from build123d import *

# Parameters (mm, degrees)
BOSS_EXTRUDE1_DEPTH = 10
SKETCH2_R           = 2
CUT_EXTRUDE1_DEPTH  = 22.973952412


with BuildPart() as part:
    # Sketch1 → Boss-Extrude1 (new body)
    with BuildSketch(Plane(origin=(0, 0, 0), x_dir=(1, 0, 0), z_dir=(0, 1, 0))):
        with BuildLine():
            Line((-5.941155294, 12.923797457), (-5.941155294, 6.423797457))
            ThreePointArc((-5.941155294, 6.423797457), (0, -8.75), (5.941155294, 6.423797457))
            Line((5.941155294, 6.423797457), (5.941155294, 12.923797457))
            Line((5.941155294, 12.923797457), (3.441155294, 12.923797457))
            Line((3.441155294, 12.923797457), (3.441155294, 8.044933203))
            Line((3.441155294, 8.044933203), (3.441155294, 6.381296909))
            ThreePointArc((3.441155294, 6.381296909), (6.22538657, 3.715785524), (7.25, 0))
            ThreePointArc((7.25, 0), (-3.715785524, -6.22538657), (-3.441155294, 6.381296909))
            Line((-3.441155294, 6.381296909), (-3.441155294, 8.044933203))
            Line((-3.441155294, 8.044933203), (-3.441155294, 12.923797457))
            Line((-3.441155294, 12.923797457), (-5.941155294, 12.923797457))
        make_face()
    extrude(amount=BOSS_EXTRUDE1_DEPTH)

    # Sketch2 → Cut-Extrude1 (cut, through all)
    with BuildSketch(Plane(origin=(5.941155294, 0, 0), x_dir=(0, 0, -1), z_dir=(1, 0, 0))):
        with Locations((9.673797457, 5)):
            Circle(SKETCH2_R)
    extrude(amount=-CUT_EXTRUDE1_DEPTH, mode=Mode.SUBTRACT)


solid = part.part
Part model, mm, in its own coordinate system. A direction names the side the tool comes from. Give positions to 0.01 mm unless a question says otherwise; leave off trailing zeros. Order: outer loops, then holes, each group sorted by start corner. A loop starts at its lowest first (then second) coordinate and runs counter-clockwise, first axis right, second up. Notation, with made-up numbers: (59.25, 17.5) - (102.25, 17.5) arc R21 cw to (102.25, 38.5) - close; hole circle Ø9 at (15, -25.75). An arc over 180 degrees is marked (long way). One line per question, with ' | ' between items.
1. Band-saw the part on A-A on x = -5.25. List the corners of the cut face in (y, z), then the cut area to 3 significant figures.
Filled in:
outline: (0, -12.92) - (10, -12.92) - (10, -5) - (0, -5) - close; (0, 5) - (10, 5) - (10, 7) - (0, 7) - close; hole circle Ø4 at (5, -9.67) | area: 86.7 mm²
2. Band-saw the part on B-B on y = 5. List the corners of the cut face in (x, z).
Filled in:
outline: (-5.94, -12.92) - (-3.44, -12.92) - (-3.44, -11.67) - (-5.94, -11.67) - close; (-5.94, -7.67) - (-3.44, -7.67) - (-3.44, -6.38) arc R7.25 cw (long way) to (3.44, -6.38) - (3.44, -7.67) - (5.94, -7.67) - (5.94, -6.42) arc R8.75 ccw (long way) to (-5.94, -6.42) - close; (3.44, -12.92) - (5.94, -12.92) - (5.94, -11.67) - (3.44, -11.67) - close
3. Drop flat-ended pins along their axis: P1, Ø5, axis at y = 5, z = -9.67, coming from the +X side; P2, Ø2, axis at y = 1, z = -6, coming from the +X side; P3, Ø2, axis at y = 4, z = -10, coming from the -X side. Give the stop position or say it passes through.
Filled in:
P1: x = 5.94 | P2: x = 7.18 | P3: x = -5.94
4. Band-saw the part on C-C on z = -10.5. List the corners of the cut face in (x, y), then the cut area to 3 significant figures.
Filled in:
outline: (-5.94, 0) - (-3.44, 0) - (-3.44, 3.18) - (-5.94, 3.18) - close; (-5.94, 6.82) - (-3.44, 6.82) - (-3.44, 10) - (-5.94, 10) - close; (3.44, 0) - (5.94, 0) - (5.94, 3.18) - (3.44, 3.18) - close; (3.44, 6.82) - (5.94, 6.82) - (5.94, 10) - (3.44, 10) - close | area: 31.8 mm²
5. Pull direction Y, two halves, no side cores. Call faces 1 (the face through (-4.674, 6.983, -9.413)), 2 (the face through (-5, 0, -6)), 3 (the face through (-5, 10, -6)): +Y half, -Y half, draft (parallel to the pull), parting line (faces both ways), or undercut.
Filled in:
face 1: undercut | face 2: -Y half | face 3: +Y half
6. Band-saw the part on D-D on x = -7. List the corners of the cut face in (y, z).
Filled in:
outline: (0, -5.25) - (10, -5.25) - (10, -1.89) - (0, -1.89) - close; (0, 1.89) - (10, 1.89) - (10, 5.25) - (0, 5.25) - close
7. Which spindle directions (+Z, -Z, +X, -X, +Y, -Y) get a long thin tool onto all of the face, cutting with end or side? Do faces 4 (the face through (5.941, 5, -7)), 5 (the face through (-5.941, 5, -12)), 6 (the face through (-3.441, 5, -12)), 7 (the face through (-5, 5, -12.924)). Say none if no direction does.
Filled in:
face 4: -Z, +X, +Y, -Y | face 5: -Z, -X, +Y, -Y | face 6: -Z, +Y, -Y | face 7: -Z, +X, -X, +Y, -Y
8. Drill centre lines: probe 1 along X at (y, z) = (3.5, 0); probe 2 along X at (y, z) = (2, -8.25); probe 3 along Z at (x, y) = (6.5, 6). Where is each one in solid material? Low to high.
Filled in:
probe 1: -8.75 to -7.25, 7.25 to 8.75 | probe 2: -5.94 to -3.44, 3.44 to 5.94 | probe 3: -5.86 to -3.21, 3.21 to 5.86
